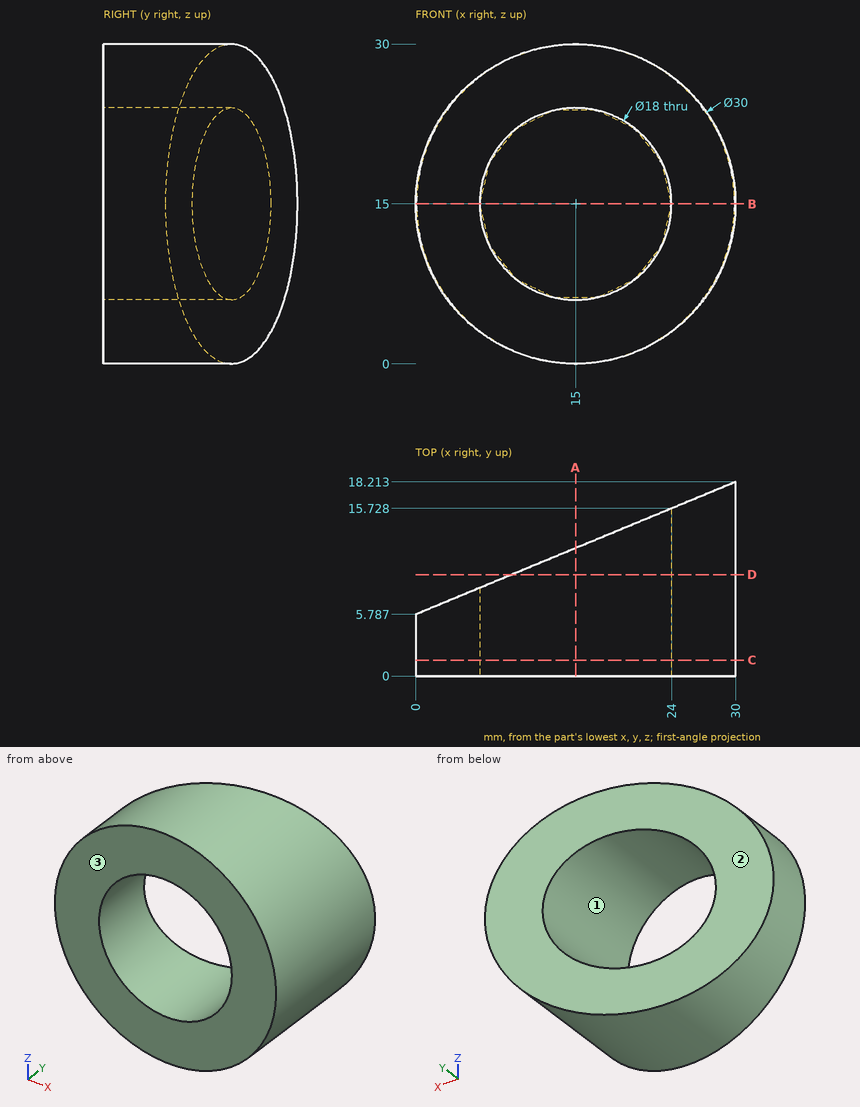
Geometry check sheet. Reference: drawing and pictorial views, mm from the part's lowest x, y, z. Round coordinates to 2 decimals unless told otherwise and drop trailing zeros. Loops run counter-clockwise (first coordinate to the right, second up) from the corner with the lowest first, then second, coordinate; pieces in that order, holes last. Notation, with made-up numbers: M 77.25,14.5 L 110.25,14.5 A26 ccw 110.25,38.5 Z; hole C 56.25,-35 d1. An arc over 180 degrees is marked long. Return JSON: item names as keys, results as strings. Group by question number.
(1) Section check D-D, the plane y = 9.5. Enter the section's corners in (x, z).
(2) Section check C-C, the plane y = 1.5. Enter the section's corners in (x, z), and give its area (3 significant figures).
(3) Mould release check, pull along X, two halves, no side actions. Record for the marked faces 1, 2 and 3: pulls with the +X half, pulls with the -X half, needs draft (parallel to the pull), parting line crosses it, or undercut.
(4) Section check B-B, the plane z = 15. Enter the section's corners in (x, y), and give its area (3 significant figures).
(5) Go/stop test with flat-tipped pins: pin 1 (5 mm diameter, centred on x = 5.5, y = 9, fed in from -Z); pin 2 (1.5 mm diameter, centred on y = 9, z = 9.5, fed in from +X); pin 3 (5 mm diameter, centred on x = 7.5, y = 4.5, fed in from +Z). Record where each tip stops, or that it passes through.
(6) Section check A-A, the plane x = 15. Enter the section's corners in (y, z), and give its area (3 significant figures).
(7) Scan lines: line 1 along Z through (x, y) = (15, 6.5); line 2 along X through (y, z) = (12, 15); line 3 along X through (y, z) = (6.5, 15). Record each from-to range of solid material in increasing order. Write a range as [from, to].
Data:
{
 "1": {"outline": "M 8.96,1.27 A15 ccw long 8.96,28.73 L 8.96,21.68 A9 cw long 8.96,8.32 Z"},
 "2": {"outline": "C 15,15 d30; hole C 15,15 d18", "area": "452 mm²"},
 "3": {"face 1": "undercut", "face 2": "pulls with the -X half", "face 3": "needs draft"},
 "4": {"outline": "M 0,0 L 6,0 L 6,8.27 L 0,5.79 Z; M 24,0 L 30,0 L 30,18.21 L 24,15.73 Z", "area": "144 mm²"},
 "5": {"pin 1": "z = 1.73", "pin 2": "x = 29.23", "pin 3": "z = 29.14"},
 "6": {"outline": "M 0,0 L 12,0 L 12,6 L 0,6 Z; M 0,24 L 12,24 L 12,30 L 0,30 Z", "area": "144 mm²"},
 "7": {"line 1": "[0, 6], [24, 30]", "line 2": "[24, 30]", "line 3": "[1.72, 6], [24, 30]"}
}
